Verification items for the finished model (mm, model axes). Give positions to 0.01 mm unless a question says otherwise; leave off trailing zeros. Write each loop counter-clockwise with the first axis right and the second up, starting at its lowest first coordinate (ties: lowest second). Pieces come first, ordered by that corner, then holes. Notation, with made-up numbers: M 89,0 L 145,0 A12 cw 145,4 Z; hole C 18,37 d2. An arc over 180 degrees is marked long. Write item = value, one per line.
from build123d import *

# Parameters (mm, degrees)
SKETCH1_R           = 75
BOSS_EXTRUDE1_DEPTH = 10
SKETCH2_R           = 16
SKETCH2_R_2         = 13
BOSS_EXTRUDE2_DEPTH = 113


with BuildPart() as part:
    # Sketch1 → Boss-Extrude1 (new body)
    with BuildSketch(Plane(origin=(0, 0, 0), x_dir=(1, 0, 0), z_dir=(0, 1, 0))):
        Circle(SKETCH1_R)
    extrude(amount=BOSS_EXTRUDE1_DEPTH)

    # Sketch2 → Boss-Extrude2 (add)
    with BuildSketch(Plane(origin=(0, 10, 0), x_dir=(1, 0, 0), z_dir=(0, 1, 0))):
        Circle(SKETCH2_R)
        Circle(SKETCH2_R_2, mode=Mode.SUBTRACT)
    extrude(amount=BOSS_EXTRUDE2_DEPTH)


solid = part.part
1) Cross-section at C-C on y = 39.5. Record the boundary of the cut face in (x, z), plus the area to 3 significant figures.
From the geometry:
outline = C 0,0 d32; hole C 0,0 d26
area = 273 mm^2
2) Depth check by flat-ended pin: P1, Ø6, axis at y = 100.5, z = -8.5, coming from the +X side (3 decimals); P2, Ø1, axis at x = -11.5, y = 34.5, coming from the +Z side; P3, Ø8, axis at x = 13, y = 50.5, coming from the +Z side. Enter the tip coordinate at first touch or a pass-through.
From the geometry:
P1 = 15.025
P2 = 11.62
P3 = 13.23
3) Cross-section at D-D on z = -41. Record the boundary of the cut face in (x, y).
From the geometry:
outline = M -62.8,0 L 62.8,0 L 62.8,10 L -62.8,10 Z
4) Draft check along Z on faces 1 (the flat face through (-1, 10, -18)), 2 (the flat face through (0, 10, 0)), 3 (the cylindrical face through (-10.316, 65.709, 7.91)), 4 (the cylindrical face through (-3.47, 65.71, 15.62)). Enter one of: +Z half, -Z half, draft (parallel to the pull), parting line (faces both ways), or undercut.
From the geometry:
face_1 = draft
face_2 = undercut
face_3 = undercut
face_4 = parting line
5) Material ranges on probe 1 along Z at (x, y) = (0, 35.5); probe 2 along Y at (x, z) = (-11.5, -52), recorded low to high. Write a range as from..to.
From the geometry:
probe_1 = -16..-13, 13..16
probe_2 = 0..10
6) Cross-section at A-A on z = 0. Record the boundary of the cut face in (x, y).
From the geometry:
outline = M -75,0 L 75,0 L 75,10 L 16,10 L 16,123 L 13,123 L 13,10 L -13,10 L -13,123 L -16,123 L -16,10 L -75,10 Z
7) Cross-section at B-B on x = 0. Record the boundary of the cut face in (y, z).
From the geometry:
outline = M 0,-75 L 10,-75 L 10,-16 L 123,-16 L 123,-13 L 10,-13 L 10,13 L 123,13 L 123,16 L 10,16 L 10,75 L 0,75 Z
